Build history of the part. All positions in model axes, mm. A direction names the side the tool comes from. Give positions to 0.01 mm unless a question says otherwise; leave off trailing zeros. Order: outer loops, then holes, each group sorted by start corner. A loop starts at its lowest first (then second) coordinate and runs counter-clockwise, first axis right, second up. Notation, with made-up numbers: (3, 45.5) - (15, 45.5) arc R19 ccw to (15, 68.5) - close; hole circle Ø10 at (87, 2.5). An arc over 180 degrees is marked (long way). Use a Markdown table: item, result. Add a question column.
(1) Wall check: line 1 (X direction, y = 9, z = -0.5); line 2 (X direction, y = 17.25, z = 0); line 3 (X direction, y = 32.2, z = 0). Give the ranges that are in metal, low to high.
(2) Which spindle directions (+Z, -Z, +X, -X, +Y, -Y) get a long thin tool onto all of the face, cutting with end or side? Do faces 1 (the face through (-0.273, 9.582, 0.14)), 2 (the face through (-12, 30, -2)). Say none if no direction does.
(3) Mould opens along Z. For faces 3 (the face through (0, 17, 10)), 4 (the face through (0, 17, -10)), 5 (the face through (-13.905, 32.535, -0.867)) say: +Z half, -Z half, draft (parallel to the pull), parting line (faces both ways), or undercut.
(4) Slice it at C-C (z = -0.5). Write the cut outline in (x, y), then the cut area to 3 significant figures.
(5) Slice it at D-D (x = 10). Write the cut outline in (y, z), then the cut area to 3 significant figures.
(6) Flat gauge pins, fed straight in: pin 1 (9 mm diameter, centred on x = -9, z = -0.5, fed in from +Y); pin 2 (4 mm diameter, centred on x = 0, y = 27.5, fed in from -Z). Where does each tip first touch, or does it go through?
(7) Slice it at B-B (x = 0). Write the cut outline in (y, z).
(8) Slice it at A-A (y = 27.5). Write the cut outline in (x, z), then the cut area to 3 significant figures.
from build123d import *

# Parameters (mm, degrees)
SKETCH1_W           = 40
SKETCH1_H           = 20
SKETCH1_R           = 2.5
BOSS_EXTRUDE1_DEPTH = 35
SKETCH2_R           = 4
CUT_EXTRUDE1_DEPTH  = 5
SKETCH3_R           = 2.1
CUT_EXTRUDE2_DEPTH  = 46


with BuildPart() as part:
    # Sketch1 → Boss-Extrude1 (new body)
    with BuildSketch(Plane(origin=(0, 0, 0), x_dir=(1, 0, 0), z_dir=(0, 1, 0))):
        Rectangle(SKETCH1_W, SKETCH1_H)
        with Locations(Location((-10, 0, 0), (0, 0, 270))):
            Circle(SKETCH1_R, mode=Mode.SUBTRACT)
        with Locations(Location((10, 0, 0), (0, 0, 270))):
            Circle(SKETCH1_R, mode=Mode.SUBTRACT)
    extrude(amount=BOSS_EXTRUDE1_DEPTH)

    # Sketch2 → Cut-Extrude1 (cut)
    with BuildSketch(Plane(origin=(0, 35, 0), x_dir=(1, 0, 0), z_dir=(0, 1, 0))):
        with Locations(Location((-10, 0, 0), (0, 0, 270))):
            Circle(SKETCH2_R)
        with Locations(Location((10, 0, 0), (0, 0, 270))):
            Circle(SKETCH2_R)
    extrude(amount=-CUT_EXTRUDE1_DEPTH, mode=Mode.SUBTRACT)

    # Sketch3 → Cut-Extrude2 (cut, through all)
    with BuildSketch(Plane.XY.offset(10)):
        with Locations((0, 27.5)):
            Circle(SKETCH3_R)
        with Locations((0, 7.5)):
            Circle(SKETCH3_R)
    extrude(amount=-CUT_EXTRUDE2_DEPTH, mode=Mode.SUBTRACT)


solid = part.part
Solution:
| question | item | result |
|---|---|---|
| 1 | line 1 | -20 to -12.45, -7.55 to -1.47, 1.47 to 7.55, 12.45 to 20 |
| 1 | line 2 | -20 to -12.5, -7.5 to 7.5, 12.5 to 20 |
| 1 | line 3 | -20 to -14, -6 to 6, 14 to 20 |
| 2 | face 1 | +Z, -Z |
| 2 | face 2 | +Y |
| 3 | face 3 | +Z half |
| 3 | face 4 | -Z half |
| 3 | face 5 | undercut |
| 4 | outline | (-20, 0) - (-12.45, 0) - (-12.45, 30) - (-13.97, 30) - (-13.97, 35) - (-20, 35) - close; (-7.55, 0) - (7.55, 0) - (7.55, 30) - (6.03, 30) - (6.03, 35) - (-6.03, 35) - (-6.03, 30) - (-7.55, 30) - close; (12.45, 0) - (20, 0) - (20, 35) - (13.97, 35) - (13.97, 30) - (12.45, 30) - close; hole circle Ø4.2 at (0, 7.5); hole circle Ø4.2 at (0, 27.5) |
| 4 | area | 999 mm2 |
| 5 | outline | (0, -10) - (35, -10) - (35, -4) - (30, -4) - (30, -2.5) - (0, -2.5) - close; (0, 2.5) - (30, 2.5) - (30, 4) - (35, 4) - (35, 10) - (0, 10) - close |
| 5 | area | 510 mm2 |
| 6 | pin 1 | y = 35 |
| 6 | pin 2 | through |
| 7 | outline | (0, -10) - (5.4, -10) - (5.4, 10) - (0, 10) - close; (9.6, -10) - (25.4, -10) - (25.4, 10) - (9.6, 10) - close; (29.6, -10) - (35, -10) - (35, 10) - (29.6, 10) - close |
| 8 | outline | (-20, -10) - (-2.1, -10) - (-2.1, 10) - (-20, 10) - close; (2.1, -10) - (20, -10) - (20, 10) - (2.1, 10) - close; hole circle Ø5 at (-10, 0); hole circle Ø5 at (10, 0) |
| 8 | area | 677 mm2 |
